Source: CAD feature listing. Evaluate the final solid. Frame: model axes, mm. A direction names the side the tool comes from. Coordinates: 2 decimals unless noted, no trailing zeros. Write each loop counter-clockwise with the first axis right and the second up, starting at its lowest first coordinate (ties: lowest second). Pieces come first, ordered by that corner, then holes. Notation, with made-up numbers: (80.25, -10.75) - (87.25, -10.75) arc R13 cw to (87.25, 1.25) - close; hole circle Ø4 at (33, 9). An arc over 180 degrees is marked (long way). One line per question, with ' | ' between items.
from build123d import *

# Parameters (mm, degrees)
BOSS_EXTRUDE1_DEPTH = 10
BOSS_EXTRUDE2_DEPTH = 40
SKETCH3_R           = 3
CUT_EXTRUDE1_DEPTH  = 134.814236911
SKETCH4_R           = 3
BOSS_EXTRUDE4_DEPTH = 20


with BuildPart() as part:
    # Sketch1 → Boss-Extrude1 (new, symmetric)
    with BuildSketch(Plane.XY):
        with BuildLine():
            Line((-40, 7.5), (-10, 7.5))
            Line((-10, 7.5), (-10, 69.587121525))
            ThreePointArc((-10, 69.587121525), (0, 117.5), (10, 69.587121525))
            Line((10, 69.587121525), (10, 7.5))
            Line((10, 7.5), (40, 7.5))
            Line((40, 7.5), (40, -7.5))
            Line((40, -7.5), (-40, -7.5))
            Line((-40, -7.5), (-40, 7.5))
        make_face()
    extrude(amount=BOSS_EXTRUDE1_DEPTH, both=True)

    # Sketch2 → Boss-Extrude2 (add)
    with BuildSketch(Plane(origin=(0, 0, 0), x_dir=(-1, 0, 0), z_dir=(0, 0, -1))):
        Polygon((-10, 7.5), (10, 7.5), (40, 7.5), (40, -7.5), (-40, -7.5), (-40, 7.5), align=None)
    extrude(amount=BOSS_EXTRUDE2_DEPTH)

    # Sketch3 → Cut-Extrude1 (cut, through all)
    with BuildSketch(Plane.XY.offset(10)):
        with Locations((0, 92.5)):
            Circle(SKETCH3_R)
    extrude(amount=-CUT_EXTRUDE1_DEPTH, mode=Mode.SUBTRACT)

    # Sketch4 → Boss-Extrude4 (add)
    with BuildSketch(Plane.XY.offset(10)):
        with BuildLine():
            ThreePointArc((-10, 69.587121525), (-23.272919558, 83.369216066), (-22.912878475, 102.5))
            Line((-22.912878475, 102.5), (-42.121373711, 93.811217193))
            ThreePointArc((-42.121373711, 93.811217193), (-47.922246908, 83.455405164), (-39.743371486, 74.853139797))
            Line((-39.743371486, 74.853139797), (-10, 69.587121525))
        make_face()
        with Locations((-38, 84.7)):
            Circle(SKETCH4_R, mode=Mode.SUBTRACT)
    extrude(amount=-BOSS_EXTRUDE4_DEPTH)


solid = part.part
Item 1: Mould query, pull axis X, two halves, no side actions, for faces 1 (the face through (-0.65, 89.57, 0.14)), 2 (the face through (-40.21, 86.73, 0.14)), 3 (the face through (40, 0, -15)), 4 (the face through (-10, 38, 0)). Classes: pulls with the +X half, pulls with the -X half, needs draft (parallel to the pull), parting line crosses it, or undercut.
Check sheet entries:
face 1: undercut | face 2: undercut | face 3: pulls with the +X half | face 4: pulls with the -X half
Item 2: Cut plane A-A on x = 0. Return loops of the section in (y, z).
Check sheet entries:
outline: (-7.5, -40) - (7.5, -40) - (7.5, -10) - (89.5, -10) - (89.5, 10) - (-7.5, 10) - close; (95.5, -10) - (117.5, -10) - (117.5, 10) - (95.5, 10) - close
Item 3: Cut plane B-B on y = 92.5. Return loops of the section in (x, z), and give its area (3 significant figures).
Check sheet entries:
outline: (-44.26, -10) - (-3, -10) - (-3, 10) - (-44.26, 10) - close; (3, -10) - (25, -10) - (25, 10) - (3, 10) - close | area: 1,270 mm²
Item 4: Cut plane C-C on z = 5. Return loops of the section in (x, y).
Check sheet entries:
outline: (-42.12, 93.81) arc R10 ccw to (-39.74, 74.85) - (-10, 69.59) - (-10, 7.5) - (-40, 7.5) - (-40, -7.5) - (40, -7.5) - (40, 7.5) - (10, 7.5) - (10, 69.59) arc R25 ccw (long way) to (-22.91, 102.5) - close; hole circle Ø6 at (-38, 84.7); hole circle Ø6 at (0, 92.5)
Item 5: Ray query, line 1 along Y through (x, z) = (-38, 4.25); line 2 along Y through (x, z) = (0, -4.75); line 3 along Y through (x, z) = (-27, -15.5). Return the intervals inside material, ascending. Write a range as [from, to].
Check sheet entries:
line 1: [-7.5, 7.5], [74.54, 81.7], [87.7, 95.68] | line 2: [-7.5, 89.5], [95.5, 117.5] | line 3: [-7.5, 7.5]
Item 6: Pin query (flat end, axial travel): pin 1 Ø3.5 at (x, y) = (-38, 84.7) entering from +Z; pin 2 Ø2 at (x, y) = (-1, 53) entering from -Z; pin 3 Ø16.5 at (y, z) = (2.5, -23.5) entering from -X; pin 4 Ø2 at (x, z) = (15.5, -22.5) entering from +Y. Return the tip coordinate at first contact, or that it passes through.
Check sheet entries:
pin 1: through | pin 2: z = -10 | pin 3: x = -40 | pin 4: y = 7.5
Item 7: Access query for faces 5 (the face through (10, 39, 0)), 6 (the face through (-4, 75, -10)), 7 (the face through (-25.08, 72.257, 0.14)), 8 (the face through (-40, 0, -15)). Directions: +Z, -Z, +X, -X, +Y, -Y. A direction counts if a zero-diameter tool reaches every point of the face in a straight line with its end or side. Return the directions, or none.
Check sheet entries:
face 5: +Z, -Z, +X | face 6: -Z, +X, -X, +Y | face 7: +Z, -Z, -X | face 8: +Z, -Z, -X, -Y
Item 8: Cut plane D-D on x = -38. Return loops of the section in (y, z).
Check sheet entries:
outline: (-7.5, -40) - (7.5, -40) - (7.5, 10) - (-7.5, 10) - close; (74.54, -10) - (81.7, -10) - (81.7, 10) - (74.54, 10) - close; (87.7, -10) - (95.68, -10) - (95.68, 10) - (87.7, 10) - close
